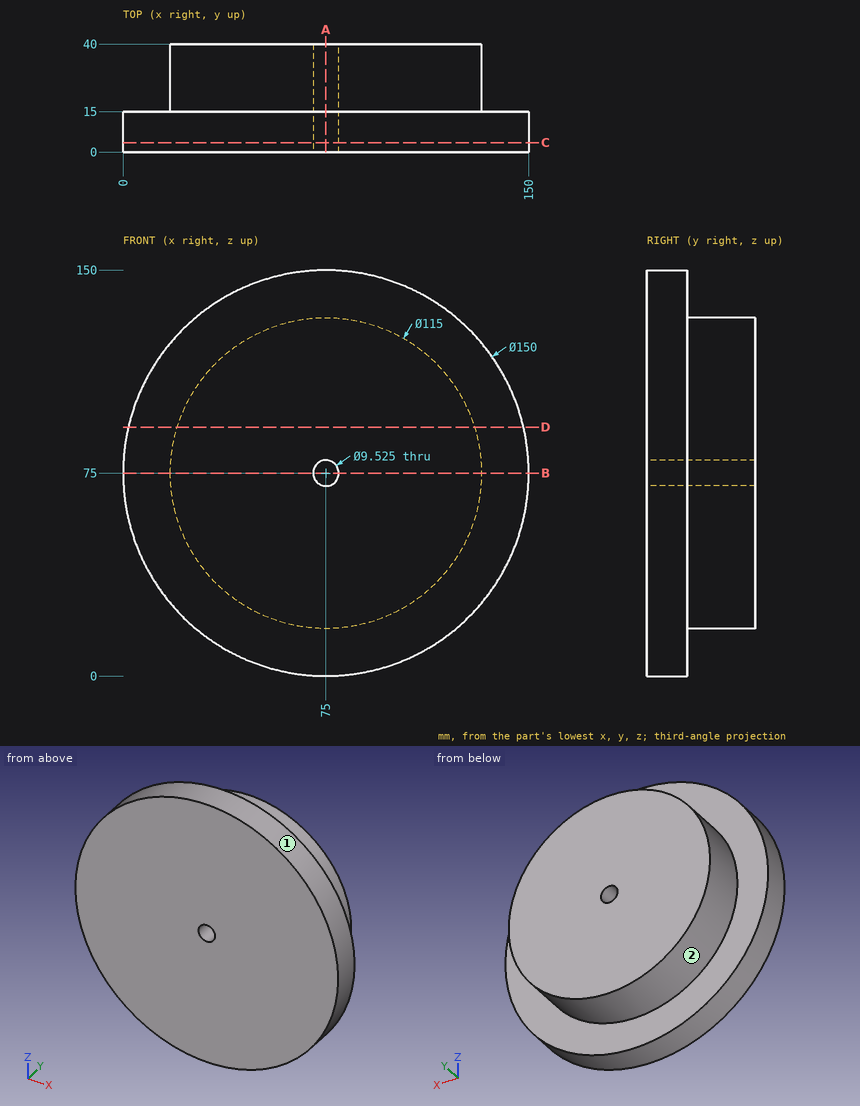
Answer from the drawing. Dimensions are ordinates in mm from the lowest x, y and z of the part. A direction names the side the tool comes from. Round coordinates to 2 decimals unless told otherwise and drop trailing zeros. Loops run counter-clockwise (first coordinate to the right, second up) from the corner with the lowest first, then second, coordinate; pieces in that order, holes last. Notation, with made-up numbers: (33, 33.5) - (67, 33.5) arc R20 ccw to (67, 37.5) - close; hole circle Ø7 at (-39, 39.25). An arc over 180 degrees is marked (long way). Return JSON: item names as keys, results as strings. Group by question number.
1. The part is cut by section D-D on z = 92. Determine the outline of the cut face in (x, y).
2. Which of the six approach directions +Z, -Z, +X, -X, +Y, -Y give full straight-line access (tool end or side, diameter ignored) to the marked faces 1 and 2?
3. The part is cut by section C-C on y = 3.5. Determine the outline of the cut face in (x, z) (1 decimal), then the cut area to 3 significant figures.
4. Consider probe 1 along Z at (x, y) = (75, 20); probe 2 along Z at (x, y) = (75, 11.5); probe 3 along Y at (x, z) = (100, 10). Determine where each line is inside the solid, lowest interval first.
5. Each of these flat-tipped pins is pushed along its axis until it touches: P1, Ø10, axis at x = 116.5, y = 16.5, coming from the +Z side; P2, Ø8, axis at y = 24, z = 19.5, coming from the -X side; P3, Ø5, axis at x = 122.5, y = 21.5, coming from the +Z side. Where does it stop, or does it pass through?
6. The part is cut by section A-A on x = 75. Determine the outline of the cut face in (y, z), then the cut area to 3 significant figures.
7. The part is cut by section B-B on z = 75. Determine the outline of the cut face in (x, y), then the cut area to 3 significant figures.
Resolved:
{
 "1": {"outline": "(1.95, 0) - (148.05, 0) - (148.05, 15) - (129.93, 15) - (129.93, 40) - (20.07, 40) - (20.07, 15) - (1.95, 15) - close"},
 "2": {"face 1": "+Y, -Y", "face 2": "+Y"},
 "3": {"outline": "circle Ø150 at (75, 75); hole circle Ø9.5 at (75, 75)", "area": "17,600 mm²"},
 "4": {"probe 1": "z = 17.5 to 70.24, 79.76 to 132.5", "probe 2": "z = 0 to 70.24, 79.76 to 150", "probe 3": "y = 0 to 15"},
 "5": {"P1": "stops at z = 140.39", "P2": "stops at x = 49.43", "P3": "stops at z = 110.79"},
 "6": {"outline": "(0, 0) - (15, 0) - (15, 17.5) - (40, 17.5) - (40, 70.24) - (0, 70.24) - close; (0, 79.76) - (40, 79.76) - (40, 132.5) - (15, 132.5) - (15, 150) - (0, 150) - close", "area": "4,740 mm²"},
 "7": {"outline": "(0, 0) - (70.24, 0) - (70.24, 40) - (17.5, 40) - (17.5, 15) - (0, 15) - close; (79.76, 0) - (150, 0) - (150, 15) - (132.5, 15) - (132.5, 40) - (79.76, 40) - close", "area": "4,740 mm²"}
}
